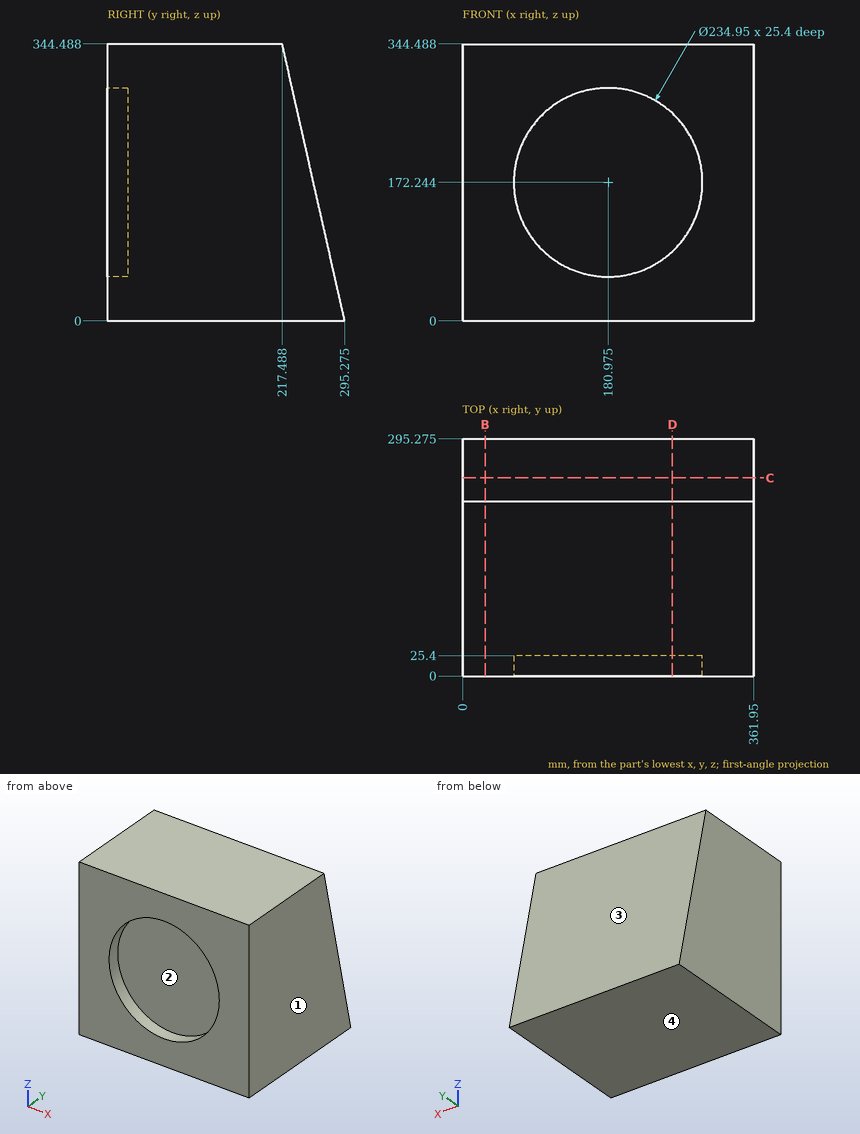
Part print with two shaded views. Sizes in mm from the minimum x, y, z corner. Coordinates: 2 decimals unless noted, no trailing zeros. Order: outer loops, then holes, each group sorted by start corner. A loop starts at its lowest first (then second) coordinate and runs counter-clockwise, first axis right, second up. Notation, with made-up numbers: M 64.5,87.25 L 113.5,87.25 A14 ccw 113.5,100.25 Z; hole C -37.75,13 d8. An arc over 180 degrees is marked long. One line per question, with ' | ' between items. Start each with the question number.
1. Flat gauge pins, fed straight in: P1, Ø10, axis at x = 193, z = 72.5, coming from the -Y side; P2, Ø5, axis at y = 254, z = 74, coming from the -X side. Where does each tip first touch, or does it go through?
2. Cut at C-C (y = 246.5). Write the cut outline in (x, z).
3. Wall check: line 1 along Y through (x, z) = (184, 151.5) (1 decimal); line 2 along Y through (x, z) = (170.5, 304). Give the ranges that are in metal, low to high. Write a range as [from, to].
4. Cut at B-B (x = 28). Write the cut outline in (y, z) (1 decimal).
5. Mould opens along Z. For the marked faces 1, 2, 3 and 4 say: +Z half, -Z half, draft (parallel to the pull), parting line (faces both ways), or undercut.
6. Cut at D-D (x = 261). Write the cut outline in (y, z) (1 decimal), plus the area to 4 significant figures.
The answers:
1) P1: stops at y = 25.4 | P2: stops at x = 0
2) outline: M 0,0 L 361.95,0 L 361.95,216 L 0,216 Z
3) line 1: y = [25.4, 261.1] | line 2: y = [0, 226.63]
4) outline: M 0,0 L 295.3,0 L 217.5,344.5 L 0,344.5 Z
5) face 1: draft | face 2: undercut | face 3: +Z half | face 4: -Z half
6) outline: M 0,0 L 295.3,0 L 217.5,344.5 L 0,344.5 L 0,258.2 L 25.4,258.2 L 25.4,86.2 L 0,86.2 Z | area: 83,950 mm2
